Part model, mm, in its own coordinate system. A direction names the side the tool comes from. Round coordinates to 2 decimals unless told otherwise and drop trailing zeros. Loops run counter-clockwise (first coordinate to the right, second up) from the corner with the lowest first, then second, coordinate; pieces in that order, holes last. Notation, with made-up numbers: M 9.25,-25.75 L 14.25,-25.75 A16 ccw 14.25,-7.75 Z; hole C -2.75,85.5 d1. An arc over 180 degrees is marked long. Write each question's results on one line, items separated by ' | '.
from build123d import *

# Parameters (mm, degrees)
ESBO_O1_W                = 40
ESBO_O1_H                = 38
ESBO_O1_W_2              = 7.5
ESBO_O1_H_2              = 2.6
RESSALTO_EXTRUS_O1_DEPTH = 10
ESBO_O1_3_W              = 2.95
ESBO_O1_3_H              = 4.4
ESBO_O3_R                = 2.45
CORTE_EXTRUS_O1_DEPTH    = 33.3
FILETE1_R                = 0.2


with BuildPart() as part:
    # Esbo_o1 → Ressalto-extrus_o1 (new body, symmetric)
    with BuildSketch(Plane.XY):
        with Locations((9.5, -19)):
            Rectangle(ESBO_O1_W, ESBO_O1_H)
        with Locations((-14.25, -7)):
            Rectangle(ESBO_O1_W_2, ESBO_O1_H_2)
        with Locations((33.25, -7)):
            Rectangle(ESBO_O1_W_2, ESBO_O1_H_2)
    extrude(amount=RESSALTO_EXTRUS_O1_DEPTH, both=True)

    # Esbo_o1_3 → Revolu_o1 (revolve)
    with BuildSketch(Plane.XY):
        with Locations((1.475, 4.2)):
            Rectangle(ESBO_O1_3_W, ESBO_O1_3_H)
        Polygon((0, 2), (0, 0), (6.8, 0), (5.85, 2), (2.95, 2), align=None)
    revolve(axis=Axis((0, 0, 0), (0, 1, 0)))

    # Esbo_o3 → Corte-extrus_o1 (cut, through all)
    with BuildSketch(Plane(origin=(0, -5.7, 0), x_dir=(1, 0, 0), z_dir=(0, 1, 0))):
        with Locations((-15.65, 4.95)):
            Circle(ESBO_O3_R)
        with Locations((-15.65, -4.95)):
            Circle(ESBO_O3_R)
        with Locations((34.65, -4.95)):
            Circle(ESBO_O3_R)
        with Locations((34.65, 4.95)):
            Circle(ESBO_O3_R)
    extrude(amount=-CORTE_EXTRUS_O1_DEPTH, mode=Mode.SUBTRACT)

    # Filete1
    filete1_edges = [part.edges().sort_by_distance(p)[0] for p in [
        (37, -7, -4.257179677),
        (37, -7, -5.642820323),
        (37, -7, 5.642820323),
        (37, -7, 4.257179677),
        (-18, -7, 5.642820323),
        (-18, -7, 4.257179677),
        (-18, -7, -4.257179677),
        (-18, -7, -5.642820323),
    ]]
    fillet(filete1_edges, radius=FILETE1_R)


solid = part.part
Item 1: Band-saw the part on D-D on y = -27. Give the cut face in (x, z), and give its area (3 significant figures).
Filled sheet:
outline: M -10.5,-10 L 29.5,-10 L 29.5,10 L -10.5,10 Z | area: 800 mm^2
Item 2: Band-saw the part on A-A on x = 34.65. Give the cut face in (y, z), and give its area (3 significant figures).
Filled sheet:
outline: M -8.3,-10 L -5.7,-10 L -5.7,-7.4 L -8.3,-7.4 Z; M -8.3,-2.5 L -5.7,-2.5 L -5.7,2.5 L -8.3,2.5 Z; M -8.3,7.4 L -5.7,7.4 L -5.7,10 L -8.3,10 Z | area: 26.5 mm^2
Item 3: Band-saw the part on B-B on z = 0. Give the cut face in (x, y), and give its area (3 significant figures).
Filled sheet:
outline: M -18,-8.3 L -10.5,-8.3 L -10.5,-38 L 29.5,-38 L 29.5,-8.3 L 37,-8.3 L 37,-5.7 L 29.5,-5.7 L 29.5,0 L 6.8,0 L 5.85,2 L 2.95,2 L 2.95,6.4 L -2.95,6.4 L -2.95,2 L -5.85,2 L -6.8,0 L -10.5,0 L -10.5,-5.7 L -18,-5.7 Z | area: 1,610 mm^2
Item 4: Wall check: L1, parallel to Z at x = -15, y = -6; L2, parallel to Y at x = 25, z = 4.5; L3, parallel to X at y = -30, z = 6.75. Give the ranges that are in metal, low to high.
Filled sheet:
L1: -10 to -7.31, -2.59 to 2.59, 7.31 to 10 | L2: -38 to 0 | L3: -10.5 to 29.5
Item 5: Which spindle directions (+Z, -Z, +X, -X, +Y, -Y) get a long thin tool onto all of the face, cutting with end or side? Do faces 1 (the flat face through (33, -5.7, 0)), 2 (the flat face through (33, -8.3, 0)), 3 (the flat face through (-14, -5.7, 0)), 4 (the flat face through (-3, 2, -1)). Say none if no direction does.
Filled sheet:
face 1: +Z, -Z, +X, +Y | face 2: +Z, -Z, +X, -Y | face 3: +Z, -Z, -X, +Y | face 4: +Y
Item 6: Drop flat-ended pins along their axis: P1, Ø2, axis at x = -14, z = 0, coming from the +Y side; P2, Ø12, axis at x = 26.5, z = -7, coming from the +Y side; P3, Ø6, axis at y = -18, z = 4.5, coming from the -X side. Give the stop position or say it passes through.
Filled sheet:
P1: y = -5.7 | P2: y = 0 | P3: x = -10.5
Item 7: Two-plate mould, pull along Z, no slides. Class faces 5 (the cylindrical face through (-2.947, 4.231, -0.13)), 6 (the cylindrical face through (-13.2, -7, 5)), 7 (the flat face through (-10.5, -3, 0)): +Z half, -Z half, draft (parallel to the pull), parting line (faces both ways), or undercut.
Filled sheet:
face 5: parting line | face 6: undercut | face 7: draft
Item 8: Band-saw the part on C-C on x = 0. Give the cut face in (y, z).
Filled sheet:
outline: M -38,-10 L 0,-10 L 0,-6.8 L 2,-5.85 L 2,-2.95 L 6.4,-2.95 L 6.4,2.95 L 2,2.95 L 2,5.85 L 0,6.8 L 0,10 L -38,10 Z
